Source: CAD feature listing. Evaluate the final solid. Frame: model axes, mm. Face numbers are marked on the shaded views. A direction names the side the tool comes from. Give positions to 0.01 mm unless a question says otherwise; leave off trailing zeros. Order: outer loops, then holes, each group sorted by start corner. A loop starts at its lowest first (then second) coordinate and runs counter-clockwise, first axis right, second up.
from build123d import *

# Parameters (mm, degrees)
F1_DEPTH = 25
F2_R     = 3
F2_R_2   = 1
F3_DEPTH = 2
F4_DEPTH = 9
F5_R     = 5
F6_DEPTH = 3


with BuildPart() as f1:
    # F0 (on Front) → F1 (new body)
    with BuildSketch(Plane.XZ):
        with BuildLine():
            Line((17.374176, 11.585681), (4.374176, 11.585681))
            ThreePointArc((4.374176, 11.585681), (0.874176, 4.085681), (4.374176, -3.414319))
            Line((4.374176, -3.414319), (17.374176, -3.414319))
            ThreePointArc((17.374176, -3.414319), (20.874176, 4.085681), (17.374176, 11.585681))
        make_face()
    extrude(amount=F1_DEPTH)

    # F2 (on face) → F3 (join)
    with BuildSketch(Plane.XZ.offset(25)):
        with Locations((10.65989, 4.085681)):
            Circle(F2_R)
        with Locations((10.65989, 4.085681)):
            Circle(F2_R_2, mode=Mode.SUBTRACT)
    extrude(amount=F3_DEPTH)

    # F2 (on face) → F4 (join)
    with BuildSketch(Plane.XZ.offset(25)):
        with Locations((10.65989, 4.085681)):
            Circle(F2_R_2)
    extrude(amount=F4_DEPTH)

    # F5 (on face) → F6 (join)
    with BuildSketch(Plane(origin=(0, 0, 0), x_dir=(-1, 0, 0), z_dir=(0, 1, 0))):
        with Locations((-10.65989, 4.085681)):
            Circle(F5_R)
    extrude(amount=F6_DEPTH)


solid = f1.part
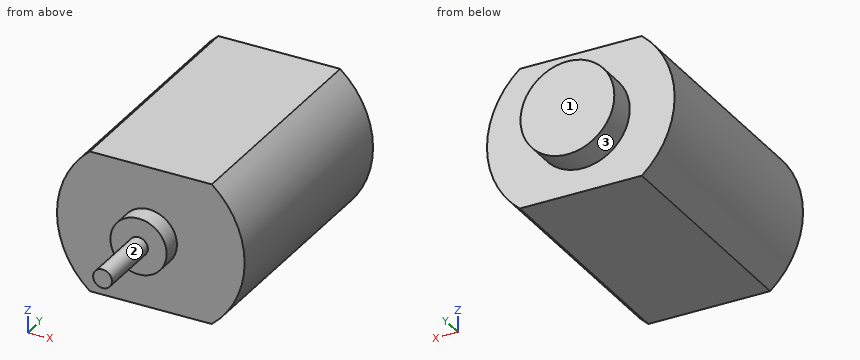
(1) Line query: line 1 along Y through (x, z) = (6.25, 0.5); line 2 along Y through (x, z) = (7.5, 3.5); line 3 along Z through (x, y) = (3.5, -3). Output: solid intervals per line, ascending.
(2) Section D-D, the plane x = 10.25. Return loops of the section in (y, z).
(3) Section A-A, the plane x = 6.25. Return loops of the section in (y, z), plus the area to 3 significant figures.
(4) Section B-B, the plane z = 1.5. Return loops of the section in (x, y).
(5) Section C-C, the plane y = -11. Return loops of the section in (x, z), plus the area to 3 significant figures.
(6) Pin query (flat end, axial travel): pin 1 Ø3 at (y, z) = (-25.5, 6) entering from +X; pin 2 Ø1 at (x, z) = (11, 7.5) entering from -Y; pin 3 Ø1.5 at (y, z) = (-4.5, 2.5) entering from -X. Return the tip coordinate at first contact, or that it passes through.
(7) Access query for the marked faces 1, 2 and 3. Directions: +Z, -Z, +X, -X, +Y, -Y. A direction counts if a zero-diameter tool reaches every point of the face in a straight line with its end or side. Return the directions, or none.
Checks:
1. line 1: y = -25 to 0
1. line 2: y = -25 to 3
1. line 3: z = -2.58 to 10.76
2. outline: (-34, 3.17) - (-27, 3.17) - (-27, 1.11) - (-25, 1.11) - (-25, -3.41) - (0, -3.41) - (0, -0.9) - (3, -0.9) - (3, 9.07) - (0, 9.07) - (0, 11.59) - (-25, 11.59) - (-25, 7.06) - (-27, 7.06) - (-27, 5) - (-34, 5) - close
3. outline: (-25, -3.41) - (0, -3.41) - (0, 1.73) - (3, 1.73) - (3, 6.44) - (0, 6.44) - (0, 11.59) - (-25, 11.59) - close
3. area: 389 mm2
4. outline: (1.22, -25) - (9.14, -25) - (9.14, -27) - (12.18, -27) - (12.18, -25) - (20.53, -25) - (20.53, 0) - (14.94, 0) - (14.94, 3) - (6.38, 3) - (6.38, 0) - (1.22, 0) - close
5. outline: (4.37, -3.41) - (17.37, -3.41) arc R9.79 ccw to (17.37, 11.59) - (4.37, 11.59) arc R9.79 ccw to start
5. area: 268 mm2
6. pin 1: stops at x = 20.86
6. pin 2: stops at y = -27
6. pin 3: stops at x = 0.91
7. face 1: +Z, -Z, +X, -X, +Y
7. face 2: -Y
7. face 3: +Y
